Build history of the part. All positions in model axes, mm. Give positions to 0.01 mm unless a question says otherwise; leave off trailing zeros. Write each loop counter-clockwise with the first axis right and the second up, starting at its lowest first coordinate (ties: lowest second). Pieces come first, ordered by that corner, then holes. Notation, with made-up numbers: (76.25, 36.5) -> (121.25, 36.5) arc R37 ccw to (121.25, 72.5) -> close; hole circle Ø6 at (48.25, -13). An arc over 180 degrees is marked (long way). Put each result on its own line as item: value.
from build123d import *

# Parameters (mm, degrees)
F1_DEPTH       = 55
F2_R           = 5
F3_R           = 9
F4_DEPTH       = 6.001
F6_D           = 4.4
F6_DEPTH       = 18
F6_CSINK_D     = 8.96
F6_CSINK_ANGLE = 90
F6_TIP         = 1.3218933619


with BuildPart() as f1:
    # F0 (on Front) → F1 (new body)
    with BuildSketch(Plane.XZ):
        Polygon((0, 6), (0, 0), (30, 0), (30, 50), (24, 50), (24, 6), align=None)
    extrude(amount=F1_DEPTH)

    # F2
    f2_edges = [f1.edges().sort_by_distance(p)[0] for p in [
        (27, -55, 50),
        (27, 0, 50),
    ]]
    fillet(f2_edges, radius=F2_R)

    # F3 (on face) → F4 (cut, through all)
    with BuildSketch(Plane(origin=(24, 0, 0), x_dir=(0, -1, 0), z_dir=(-1, 0, 0))):
        with Locations((27.5, 27)):
            Circle(F3_R)
    extrude(amount=-F4_DEPTH, mode=Mode.SUBTRACT)

    # F6
    with Locations(Plane.XY.offset(6)):
        with Locations((6, -6), (18, -49)):
            CounterSinkHole(F6_D / 2, F6_CSINK_D / 2, depth=F6_DEPTH, counter_sink_angle=F6_CSINK_ANGLE)
            with Locations((0, 0, -(F6_DEPTH + F6_TIP / 2))):  # 118° drill point
                Cone(0, F6_D / 2, F6_TIP, mode=Mode.SUBTRACT)


solid = f1.part
1) Wall check: L1, parallel to X at y = -6, z = 1.6; L2, parallel to Y at x = 18, z = 1.9; L3, parallel to Z at x = 25.5, y = -27.5. Give the ranges that are in metal, low to high.
Filled sheet:
L1: 0 to 3.8, 8.2 to 30
L2: -55 to -51.2, -46.8 to 0
L3: 0 to 18, 36 to 50
2) Pin check, flat tip, straight feed: pin 1 (7 mm diameter, centred on x = 7, y = -34, fed in from +Z). Stop position of the tip, or through.
Filled sheet:
pin 1: z = 6
3) Slice it at B-B (z = 27). Write the cut outline in (x, y).
Filled sheet:
outline: (24, -55) -> (30, -55) -> (30, -36.5) -> (24, -36.5) -> close; (24, -18.5) -> (30, -18.5) -> (30, 0) -> (24, 0) -> close
4) Slice it at C-C (y = -6). Write the cut outline in (x, z), plus the area to 3 significant figures.
Filled sheet:
outline: (0, 0) -> (3.8, 0) -> (3.8, 3.72) -> (1.52, 6) -> (0, 6) -> close; (8.2, 0) -> (30, 0) -> (30, 50) -> (24, 50) -> (24, 6) -> (10.48, 6) -> (8.2, 3.72) -> close
area: 412 mm2
5) Slice it at A-A (y = -27.5). Write the cut outline in (x, z), plus the area to 3 significant figures.
Filled sheet:
outline: (0, 0) -> (30, 0) -> (30, 18) -> (24, 18) -> (24, 6) -> (0, 6) -> close; (24, 36) -> (30, 36) -> (30, 50) -> (24, 50) -> close
area: 336 mm2
6) Slice it at D-D (z = 22). Write the cut outline in (x, y), plus the area to 3 significant figures.
Filled sheet:
outline: (24, -55) -> (30, -55) -> (30, -34.98) -> (24, -34.98) -> close; (24, -20.02) -> (30, -20.02) -> (30, 0) -> (24, 0) -> close
area: 240 mm2
7) Pull direction Z, two halves, no side cores. Call faces 1 (the cylindrical face through (26.96, -32.34, 34.59)), 2 (the flat face through (12, -27, 6)), 3 (the flat face through (24, -27, 38)), 4 (the flat face through (15, -27, 0)): released by +Z, released by -Z, zero draft, split by the parting line, or undercut.
Filled sheet:
face 1: undercut
face 2: released by +Z
face 3: zero draft
face 4: released by -Z
